```python
from build123d import *

# Parameters (mm, degrees)
F0_W     = 45
F0_H     = 55
F1_DEPTH = 10
F3_DEPTH = 7
F4_W     = 16
F4_H     = 3
F5_DEPTH = 55.0010001


with BuildPart() as f1:
    # F0 (on Front) → F1 (new body)
    with BuildSketch(Plane.XZ):
        Rectangle(F0_W, F0_H)
    extrude(amount=F1_DEPTH)

    # F2 (on face) → F3 (cut)
    with BuildSketch(Plane.XZ.offset(10)):
        with BuildLine():
            Line((3.9123152383, -27.5), (3.9123152383, 0))
            add(Edge.make_bspline(
                [(3.9123152383, 0), (4.5414378197, 20.6852698078), (10.9457386037, 10.2673236529), (11.484915749, 27.5)],
                knots=[0, 0, 0, 0, 28.5235740835, 28.5235740835, 28.5235740835, 28.5235740835], degree=3))
            Line((11.484915749, 27.5), (-11.484915749, 27.5))
            add(Edge.make_bspline(
                [(-3.9123152383, 0), (-4.5414378197, 20.6852698078), (-10.9457386037, 10.2673236529), (-11.484915749, 27.5)],
                knots=[0, 0, 0, 0, 28.5235740835, 28.5235740835, 28.5235740835, 28.5235740835], degree=3))
            Line((-3.9123152383, 0), (-3.9123152383, -27.5))
            Line((-3.9123152383, -27.5), (0, -27.5))
            Line((0, -27.5), (3.9123152383, -27.5))
        make_face()
    extrude(amount=-F3_DEPTH, mode=Mode.SUBTRACT)

    # F4 (on face) → F5 (cut, through all)
    with BuildSketch(Plane.XY.offset(27.5)):
        with Locations((0, -4.5)):
            Rectangle(F4_W, F4_H)
    extrude(amount=-F5_DEPTH, mode=Mode.SUBTRACT)


solid = f1.part
```
Here's how the part is built. I have some questions about the finished solid (model axes, mm). A direction names the side the tool comes from. Coordinates: 2 decimals unless noted, no trailing zeros. Loops run counter-clockwise (first coordinate to the right, second up) from the corner with the lowest first, then second, coordinate; pieces in that order, holes last. Notation, with made-up numbers: (36, 54) - (47, 54) arc R27 cw to (47, 87) - close; hole circle Ø5 at (86, -4.75). An arc over 180 degrees is marked (long way). Answer as CSV lines item,"result".
Q1. For faces 4 (the face through (-22.5, -5, 0)), 5 (the face through (-3.912, -8, -14)), 6 (the face through (6, -6, -6)), which set-ups out of +Z, -Z, +X, -X, +Y, -Y let a thin tool reach every point of the face, with its end or its side?
Response:
face 4,"+Z, -Z, -X, +Y, -Y"
face 5,"+Z, -Z, -Y"
face 6,"+Z, -Z"
Q2. We'd pull the mould along X, two halves only. Please class faces 1 (the face through (-13, -10, 0)), 2 (the face through (22.5, -5, 0)), 3 (the face through (0, -3, 0)): pulls with the +X half, pulls with the -X half, needs draft (parallel to the pull), parting line crosses it, or undercut.
Response:
face 1,"needs draft"
face 2,"pulls with the +X half"
face 3,"undercut"
Q3. If we section it at A-A, the plane z = -7: Write out the boundary of the cut face in (x, y), and give its area (3 significant figures).
Response:
outline,"(-22.5, -10) - (-3.91, -10) - (-3.91, -6) - (-8, -6) - (-8, -3) - (8, -3) - (8, -6) - (3.91, -6) - (3.91, -10) - (22.5, -10) - (22.5, 0) - (-22.5, 0) - close"
area,"371 mm2"
Q4. If I drill on L1, parallel to X at y = -5.75, z = 0; L2, parallel to X at y = -7.75, z = -21; L3, parallel to Y at x = -2, z = 16, over which ranges is the centre line in solid material (lowest first)? Write a range as [from, to].
Response:
L1,"[-22.5, -8], [8, 22.5]"
L2,"[-22.5, -3.91], [3.91, 22.5]"
L3,"[-3, 0]"
Q5. If we section it at B-B, the plane x = 0: Write out the boundary of the cut face in (y, z), and give its area (3 significant figures).
Response:
outline,"(-3, -27.5) - (0, -27.5) - (0, 27.5) - (-3, 27.5) - close"
area,"165 mm2"
